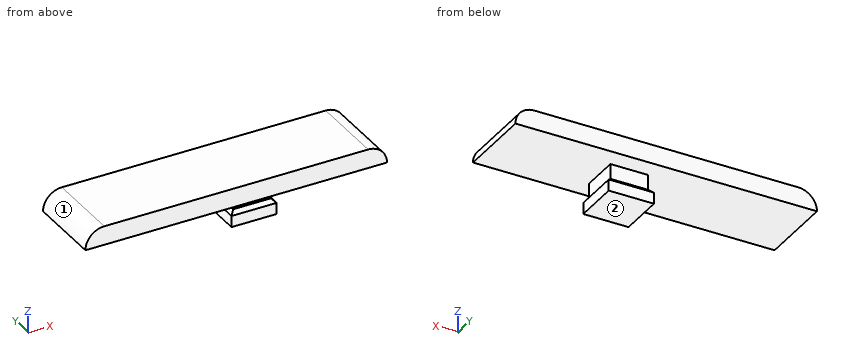
```python
from build123d import *

# Parameters (mm, degrees)
F0_W          = 101.6
F0_H          = 25.4
F0_W_2        = 12.7
F0_H_2        = 12.7
F1_DEPTH      = 6.35
F2_R          = 6.34999
F3_R          = 6.34999
F4_DEPTH      = 3.81
F5_W          = 15.24
F5_H          = 15.24
F5_W_2        = 12.7
F5_H_2        = 12.7
F6_DEPTH      = 6.35
F7_T4_DEPTH   = 28.3041495789
F7_T10_DEPTH  = 28.3041495789
F7_T16_DEPTH  = 28.3041495789
F7_T23_DEPTH  = 28.3041495789
F7_T29_DEPTH  = 28.3041495789
F7_T35_DEPTH  = 28.3041495789
F7_T41_DEPTH  = 28.3041495789
F7_T47_DEPTH  = 28.3041495789
F7_T54_DEPTH  = 28.3041495789
F7_T60_DEPTH  = 28.3041495789
F7_T66_DEPTH  = 28.3041495789
F7_T72_DEPTH  = 28.3041495789
F7_T78_DEPTH  = 28.3041495789
F7_T85_DEPTH  = 28.3041495789
F7_T91_DEPTH  = 28.3041495789
F7_T97_DEPTH  = 28.3041495789
F7_T103_DEPTH = 28.3041495789
F7_T109_DEPTH = 28.3041495789
F7_T116_DEPTH = 28.3041495789
F7_T122_DEPTH = 28.3041495789


# Not quite as in the source:
# - a fillet or chamfer that OpenCascade refuses, or shapes differently, is made with other operations: its cross-section is extruded or revolved along the edge and cut away or added
# - a fillet or chamfer is up to 0.001 mm smaller than in the source, because OpenCascade refuses the exact size


with BuildPart() as f1:
    # F0 (on Top) → F1 (new body)
    with BuildSketch(Plane.XY):
        Rectangle(F0_W, F0_H)
        with Locations((8.89, 0)):
            Rectangle(F0_W_2, F0_H_2, mode=Mode.SUBTRACT)
        with Locations((8.89, 0)):
            Rectangle(F0_W_2, F0_H_2)
    extrude(amount=F1_DEPTH)

    # F2 (radius 6.35 in the source; OpenCascade refuses exactly that, so slightly less here)
    f2_edges = [f1.edges().sort_by_distance(p)[0] for p in [
        (-50.8, 0, 6.35),
    ]]
    fillet(f2_edges, radius=F2_R)

    # F3 (radius 6.35 in the source; OpenCascade refuses exactly that, so slightly less here)
    f3_edges = [f1.edges().sort_by_distance(p)[0] for p in [
        (50.8, 0, 6.35),
    ]]
    fillet(f3_edges, radius=F3_R)

    # F0 (on Top) → F4 (join)
    with BuildSketch(Plane.XY):
        with Locations((8.89, 0)):
            Rectangle(F0_W_2, F0_H_2)
    extrude(amount=-F4_DEPTH)

    # F5 (on face) → F6 (join)
    with BuildSketch(Plane(origin=(0, 0, -3.81), x_dir=(1, 0, 0), z_dir=(0, 0, -1))):
        with Locations((8.89, 0)):
            Rectangle(F5_W, F5_H)
        with Locations((8.89, 0)):
            Rectangle(F5_W_2, F5_H_2, mode=Mode.SUBTRACT)
        with Locations((8.89, 0)):
            Rectangle(F5_W_2, F5_H_2)
    extrude(amount=F6_DEPTH)

    # F7: chamfer of 2.54 on 4 edges, made by hand


with BuildPart() as f7_tool2:
    # F7_s3 → F7_t4 (new body)
    with BuildSketch(Plane.XZ.offset(14.1520747894)):
        Polygon((1.27, -6.35), (3.81, -3.81), (1.27, -3.81), align=None)
    extrude(amount=-F7_T4_DEPTH)

    split(bisect_by=Plane.XZ.offset(6.35), keep=Keep.TOP)

    split(bisect_by=Plane.YZ.offset(2.54), keep=Keep.BOTTOM)


with BuildPart() as f1_1:
    add(f1.part)

    # F7_t1: cut F7_tool2
    add(f7_tool2.part, mode=Mode.SUBTRACT)


with BuildPart() as f7_tool8:
    # F7_s9 → F7_t10 (new body)
    with BuildSketch(Plane.XZ.offset(14.1520747894)):
        Polygon((1.27, -6.35), (3.81, -3.81), (1.27, -3.81), align=None)
    extrude(amount=-F7_T10_DEPTH)

    split(bisect_by=Plane.XZ.offset(6.35), keep=Keep.TOP)

    split(bisect_by=Plane.YZ.offset(2.54), keep=Keep.TOP)


with BuildPart() as f1_2:
    add(f1_1.part)

    # F7_t7: cut F7_tool8
    add(f7_tool8.part, mode=Mode.SUBTRACT)


with BuildPart() as f7_tool14:
    # F7_s15 → F7_t16 (new body)
    with BuildSketch(Plane.XZ.offset(14.1520747894)):
        Polygon((1.27, -6.35), (3.81, -3.81), (1.27, -3.81), align=None)
    extrude(amount=-F7_T16_DEPTH)

    split(bisect_by=Plane.XZ.offset(6.35), keep=Keep.BOTTOM)

    split(bisect_by=Plane.YZ.offset(2.54), keep=Keep.BOTTOM)

    split(bisect_by=Plane.XZ.offset(-6.35), keep=Keep.TOP)


with BuildPart() as f1_3:
    add(f1_2.part)

    # F7_t13: cut F7_tool14
    add(f7_tool14.part, mode=Mode.SUBTRACT)


with BuildPart() as f7_tool21:
    # F7_s22 → F7_t23 (new body)
    with BuildSketch(Plane.XZ.offset(14.1520747894)):
        Polygon((1.27, -6.35), (3.81, -3.81), (1.27, -3.81), align=None)
    extrude(amount=-F7_T23_DEPTH)

    split(bisect_by=Plane.YZ.offset(2.54), keep=Keep.BOTTOM)

    split(bisect_by=Plane.XZ.offset(-6.35), keep=Keep.BOTTOM)


with BuildPart() as f1_4:
    add(f1_3.part)

    # F7_t20: cut F7_tool21
    add(f7_tool21.part, mode=Mode.SUBTRACT)


with BuildPart() as f7_tool27:
    # F7_s28 → F7_t29 (new body)
    with BuildSketch(Plane.XZ.offset(14.1520747894)):
        Polygon((1.27, -6.35), (3.81, -3.81), (1.27, -3.81), align=None)
    extrude(amount=-F7_T29_DEPTH)

    split(bisect_by=Plane.YZ.offset(2.54), keep=Keep.TOP)

    split(bisect_by=Plane.XZ.offset(-6.35), keep=Keep.BOTTOM)


with BuildPart() as f1_5:
    add(f1_4.part)

    # F7_t26: cut F7_tool27
    add(f7_tool27.part, mode=Mode.SUBTRACT)


with BuildPart() as f7_tool33:
    # F7_s34 → F7_t35 (new body)
    with BuildSketch(Plane.YZ.offset(23.0420747894)):
        Polygon((-5.08, -3.81), (-7.62, -6.35), (-7.62, -3.81), align=None)
    extrude(amount=-F7_T35_DEPTH)

    split(bisect_by=Plane.YZ.offset(15.24), keep=Keep.TOP)

    split(bisect_by=Plane.XZ.offset(6.35), keep=Keep.BOTTOM)


with BuildPart() as f1_6:
    add(f1_5.part)

    # F7_t32: cut F7_tool33
    add(f7_tool33.part, mode=Mode.SUBTRACT)


with BuildPart() as f7_tool39:
    # F7_s40 → F7_t41 (new body)
    with BuildSketch(Plane.YZ.offset(23.0420747894)):
        Polygon((-5.08, -3.81), (-7.62, -6.35), (-7.62, -3.81), align=None)
    extrude(amount=-F7_T41_DEPTH)

    split(bisect_by=Plane.YZ.offset(15.24), keep=Keep.TOP)

    split(bisect_by=Plane.XZ.offset(6.35), keep=Keep.TOP)


with BuildPart() as f1_7:
    add(f1_6.part)

    # F7_t38: cut F7_tool39
    add(f7_tool39.part, mode=Mode.SUBTRACT)


with BuildPart() as f7_tool45:
    # F7_s46 → F7_t47 (new body)
    with BuildSketch(Plane.YZ.offset(23.0420747894)):
        Polygon((-5.08, -3.81), (-7.62, -6.35), (-7.62, -3.81), align=None)
    extrude(amount=-F7_T47_DEPTH)

    split(bisect_by=Plane.YZ.offset(15.24), keep=Keep.BOTTOM)

    split(bisect_by=Plane.XZ.offset(6.35), keep=Keep.TOP)

    split(bisect_by=Plane.YZ.offset(2.54), keep=Keep.TOP)


with BuildPart() as f1_8:
    add(f1_7.part)

    # F7_t44: cut F7_tool45
    add(f7_tool45.part, mode=Mode.SUBTRACT)


with BuildPart() as f7_tool52:
    # F7_s53 → F7_t54 (new body)
    with BuildSketch(Plane.YZ.offset(23.0420747894)):
        Polygon((-5.08, -3.81), (-7.62, -6.35), (-7.62, -3.81), align=None)
    extrude(amount=-F7_T54_DEPTH)

    split(bisect_by=Plane.XZ.offset(6.35), keep=Keep.BOTTOM)

    split(bisect_by=Plane.YZ.offset(2.54), keep=Keep.BOTTOM)


with BuildPart() as f1_9:
    add(f1_8.part)

    # F7_t51: cut F7_tool52
    add(f7_tool52.part, mode=Mode.SUBTRACT)


with BuildPart() as f7_tool58:
    # F7_s59 → F7_t60 (new body)
    with BuildSketch(Plane.YZ.offset(23.0420747894)):
        Polygon((-5.08, -3.81), (-7.62, -6.35), (-7.62, -3.81), align=None)
    extrude(amount=-F7_T60_DEPTH)

    split(bisect_by=Plane.XZ.offset(6.35), keep=Keep.TOP)

    split(bisect_by=Plane.YZ.offset(2.54), keep=Keep.BOTTOM)


with BuildPart() as f1_10:
    add(f1_9.part)

    # F7_t57: cut F7_tool58
    add(f7_tool58.part, mode=Mode.SUBTRACT)


with BuildPart() as f7_tool64:
    # F7_s65 → F7_t66 (new body)
    with BuildSketch(Plane.XZ.offset(-14.1520747894)):
        Polygon((16.51, -6.35), (13.97, -3.81), (16.51, -3.81), align=None)
    extrude(amount=F7_T66_DEPTH)

    split(bisect_by=Plane.YZ.offset(15.24), keep=Keep.TOP)

    split(bisect_by=Plane.XZ.offset(-6.35), keep=Keep.BOTTOM)


with BuildPart() as f1_11:
    add(f1_10.part)

    # F7_t63: cut F7_tool64
    add(f7_tool64.part, mode=Mode.SUBTRACT)


with BuildPart() as f7_tool70:
    # F7_s71 → F7_t72 (new body)
    with BuildSketch(Plane.XZ.offset(-14.1520747894)):
        Polygon((16.51, -6.35), (13.97, -3.81), (16.51, -3.81), align=None)
    extrude(amount=F7_T72_DEPTH)

    split(bisect_by=Plane.YZ.offset(15.24), keep=Keep.BOTTOM)

    split(bisect_by=Plane.XZ.offset(-6.35), keep=Keep.BOTTOM)


with BuildPart() as f1_12:
    add(f1_11.part)

    # F7_t69: cut F7_tool70
    add(f7_tool70.part, mode=Mode.SUBTRACT)


with BuildPart() as f7_tool76:
    # F7_s77 → F7_t78 (new body)
    with BuildSketch(Plane.XZ.offset(-14.1520747894)):
        Polygon((16.51, -6.35), (13.97, -3.81), (16.51, -3.81), align=None)
    extrude(amount=F7_T78_DEPTH)

    split(bisect_by=Plane.YZ.offset(15.24), keep=Keep.TOP)

    split(bisect_by=Plane.XZ.offset(6.35), keep=Keep.BOTTOM)

    split(bisect_by=Plane.XZ.offset(-6.35), keep=Keep.TOP)


with BuildPart() as f1_13:
    add(f1_12.part)

    # F7_t75: cut F7_tool76
    add(f7_tool76.part, mode=Mode.SUBTRACT)


with BuildPart() as f7_tool83:
    # F7_s84 → F7_t85 (new body)
    with BuildSketch(Plane.XZ.offset(-14.1520747894)):
        Polygon((16.51, -6.35), (13.97, -3.81), (16.51, -3.81), align=None)
    extrude(amount=F7_T85_DEPTH)

    split(bisect_by=Plane.YZ.offset(15.24), keep=Keep.TOP)

    split(bisect_by=Plane.XZ.offset(6.35), keep=Keep.TOP)


with BuildPart() as f1_14:
    add(f1_13.part)

    # F7_t82: cut F7_tool83
    add(f7_tool83.part, mode=Mode.SUBTRACT)


with BuildPart() as f7_tool89:
    # F7_s90 → F7_t91 (new body)
    with BuildSketch(Plane.XZ.offset(-14.1520747894)):
        Polygon((16.51, -6.35), (13.97, -3.81), (16.51, -3.81), align=None)
    extrude(amount=F7_T91_DEPTH)

    split(bisect_by=Plane.YZ.offset(15.24), keep=Keep.BOTTOM)

    split(bisect_by=Plane.XZ.offset(6.35), keep=Keep.TOP)


with BuildPart() as f1_15:
    add(f1_14.part)

    # F7_t88: cut F7_tool89
    add(f7_tool89.part, mode=Mode.SUBTRACT)


with BuildPart() as f7_tool95:
    # F7_s96 → F7_t97 (new body)
    with BuildSketch(Plane.YZ.offset(-5.2620747894)):
        Polygon((7.62, -6.35), (5.08, -3.81), (7.62, -3.81), align=None)
    extrude(amount=F7_T97_DEPTH)

    split(bisect_by=Plane.YZ.offset(2.54), keep=Keep.BOTTOM)

    split(bisect_by=Plane.XZ.offset(-6.35), keep=Keep.BOTTOM)


with BuildPart() as f1_16:
    add(f1_15.part)

    # F7_t94: cut F7_tool95
    add(f7_tool95.part, mode=Mode.SUBTRACT)


with BuildPart() as f7_tool101:
    # F7_s102 → F7_t103 (new body)
    with BuildSketch(Plane.YZ.offset(-5.2620747894)):
        Polygon((7.62, -6.35), (5.08, -3.81), (7.62, -3.81), align=None)
    extrude(amount=F7_T103_DEPTH)

    split(bisect_by=Plane.YZ.offset(2.54), keep=Keep.BOTTOM)

    split(bisect_by=Plane.XZ.offset(-6.35), keep=Keep.TOP)


with BuildPart() as f1_17:
    add(f1_16.part)

    # F7_t100: cut F7_tool101
    add(f7_tool101.part, mode=Mode.SUBTRACT)


with BuildPart() as f7_tool107:
    # F7_s108 → F7_t109 (new body)
    with BuildSketch(Plane.YZ.offset(-5.2620747894)):
        Polygon((7.62, -6.35), (5.08, -3.81), (7.62, -3.81), align=None)
    extrude(amount=F7_T109_DEPTH)

    split(bisect_by=Plane.YZ.offset(15.24), keep=Keep.BOTTOM)

    split(bisect_by=Plane.YZ.offset(2.54), keep=Keep.TOP)

    split(bisect_by=Plane.XZ.offset(-6.35), keep=Keep.BOTTOM)


with BuildPart() as f1_18:
    add(f1_17.part)

    # F7_t106: cut F7_tool107
    add(f7_tool107.part, mode=Mode.SUBTRACT)


with BuildPart() as f7_tool114:
    # F7_s115 → F7_t116 (new body)
    with BuildSketch(Plane.YZ.offset(-5.2620747894)):
        Polygon((7.62, -6.35), (5.08, -3.81), (7.62, -3.81), align=None)
    extrude(amount=F7_T116_DEPTH)

    split(bisect_by=Plane.YZ.offset(15.24), keep=Keep.TOP)

    split(bisect_by=Plane.XZ.offset(-6.35), keep=Keep.BOTTOM)


with BuildPart() as f1_19:
    add(f1_18.part)

    # F7_t113: cut F7_tool114
    add(f7_tool114.part, mode=Mode.SUBTRACT)


with BuildPart() as f7_tool120:
    # F7_s121 → F7_t122 (new body)
    with BuildSketch(Plane.YZ.offset(-5.2620747894)):
        Polygon((7.62, -6.35), (5.08, -3.81), (7.62, -3.81), align=None)
    extrude(amount=F7_T122_DEPTH)

    split(bisect_by=Plane.YZ.offset(15.24), keep=Keep.TOP)

    split(bisect_by=Plane.XZ.offset(-6.35), keep=Keep.TOP)


with BuildPart() as f1_20:
    add(f1_19.part)

    # F7_t119: cut F7_tool120
    add(f7_tool120.part, mode=Mode.SUBTRACT)


solid = f1_20.part
```
Here's how the part is built. I have some questions about the finished solid (model axes, mm). Face numbers are marked on the shaded views. Round coordinates to 2 decimals unless told otherwise and drop trailing zeros. Order: outer loops, then holes, each group sorted by start corner. A loop starts at its lowest first (then second) coordinate and runs counter-clockwise, first axis right, second up. Notation, with made-up numbers: M 27,-14 L 53,-14 A21 cw 53,14 Z; hole C 17,71.25 d2. An arc over 180 degrees is marked long. Answer in a Markdown table with one row per item.
Item 1: Imagine slicing it at A-A, the plane x = 9. Write out the boundary of the cut face in (y, z).
A:
| item | result |
|---|---|
| outline | M -12.7,0 L -6.35,0 L -6.35,-5.08 L -7.62,-6.35 L -7.62,-10.16 L 7.62,-10.16 L 7.62,-6.35 L 6.35,-5.08 L 6.35,0 L 12.7,0 L 12.7,6.35 L -12.7,6.35 Z |
Item 2: If I drill on L1, parallel to Y at x = 13.5, z = -8.75; L2, parallel to Z at x = 13, y = 8; L3, parallel to Y at x = 12.5, z = -1, over which ranges is the centre line in solid material (lowest first)? Write a range as from..to.
A:
| item | result |
|---|---|
| L1 | y = -7.62..7.62 |
| L2 | z = 0..6.35 |
| L3 | y = -6.35..6.35 |
Item 3: Imagine slicing it at C-C, the plane z = -2.5. Write out the boundary of the cut face in (x, y).
A:
| item | result |
|---|---|
| outline | M 2.54,-6.35 L 15.24,-6.35 L 15.24,6.35 L 2.54,6.35 Z |
Item 4: I'm going to push flat-ended pins straight in: pin 1 (1.9 mm diameter, centred on y = -2, z = -8, fed in from +X); pin 2 (1.5 mm diameter, centred on y = -2, z = -2.5, fed in from -X); pin 3 (10 mm diameter, centred on x = -1, y = -3.5, fed in from -Z); pin 4 (4 mm diameter, centred on y = -2.5, z = -3.5, fed in from +X). Where does each tip first touch, or does it pass through?
A:
| item | result |
|---|---|
| pin 1 | stops at x = 16.51 |
| pin 2 | stops at x = 2.54 |
| pin 3 | stops at z = -10.16 |
| pin 4 | stops at x = 15.66 |
Item 5: Thinking about a two-plate mould opening in X: for the marked faces 1 and 2, which applies, +X half, -X half, draft (parallel to the pull), parting line (faces both ways), or undercut?
A:
| item | result |
|---|---|
| face 1 | -X half |
| face 2 | draft |
